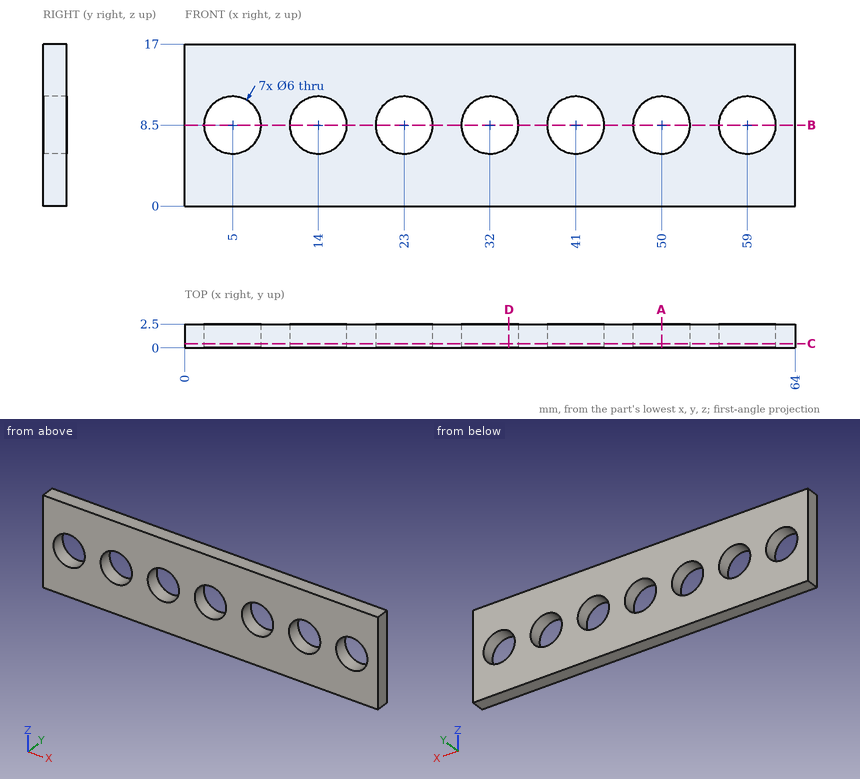
Job drawing, mm, ordinate dimensions from the low corner. One solid piece. Give positions to 0.01 mm unless a question says otherwise; leave off trailing zeros. Loops run counter-clockwise (first coordinate to the right, second up) from the corner with the lowest first, then second, coordinate; pieces in that order, holes last. Notation, with made-up numbers: (61.5, -27) -> (119.5, -27) arc R16 ccw to (119.5, -8) -> close; hole circle Ø8 at (14.5, 55.5). An arc over 180 degrees is marked (long way). Use a Markdown table: item, result. Add a question column.
(1) Slice it at A-A on x = 50. List the corners of the cut face in (y, z).
(2) Slice it at C-C on y = 0.45. List the corners of the cut face in (x, z), and give its area (3 significant figures).
(3) Slice it at D-D on x = 34. List the corners of the cut face in (y, z).
(4) Drop flat-ended pins along their axis: pin 1 Ø5 at (x, z) = (41, 8.5) entering from -Y (1 decimal); pin 2 Ø2 at (x, z) = (9.5, 14) entering from -Y. Give the stop position or say it passes through.
(5) Wall check: line 1 along Z through (x, y) = (38.5, 0.8); line 2 along Z through (x, y) = (50.5, 0.3). Give the ranges that are in metal, low to high.
(6) Slice it at B-B on z = 8.5. Give the number of separate pieces and of enclosed holes in the cut face, and give its area (3 significant figures).
Filled sheet:
| question | item | result |
|---|---|---|
| 1 | outline | (0, 0) -> (2.5, 0) -> (2.5, 5.5) -> (0, 5.5) -> close; (0, 11.5) -> (2.5, 11.5) -> (2.5, 17) -> (0, 17) -> close |
| 2 | outline | (0, 0) -> (64, 0) -> (64, 17) -> (0, 17) -> close; hole circle Ø6 at (5, 8.5); hole circle Ø6 at (14, 8.5); hole circle Ø6 at (23, 8.5); hole circle Ø6 at (32, 8.5); hole circle Ø6 at (41, 8.5); hole circle Ø6 at (50, 8.5); hole circle Ø6 at (59, 8.5) |
| 2 | area | 890 mm2 |
| 3 | outline | (0, 0) -> (2.5, 0) -> (2.5, 6.26) -> (0, 6.26) -> close; (0, 10.74) -> (2.5, 10.74) -> (2.5, 17) -> (0, 17) -> close |
| 4 | pin 1 | through |
| 4 | pin 2 | y = 0 |
| 5 | line 1 | 0 to 6.84, 10.16 to 17 |
| 5 | line 2 | 0 to 5.54, 11.46 to 17 |
| 6 | separate pieces | 8 |
| 6 | enclosed holes | 0 |
| 6 | area | 55.0 mm2 |
